Check sheet for the modelled part. Datum: model origin and axes. Units: mm. A direction names the side the tool comes from. Coordinates: 2 decimals unless noted, no trailing zeros. Loops run counter-clockwise (first coordinate to the right, second up) from the corner with the lowest first, then second, coordinate; pieces in that order, holes last.
from build123d import *

# Parameters (mm, degrees)
SKETCH1_R           = 32.75
BOSS_EXTRUDE1_DEPTH = 80.75
SKETCH12_R          = 6
BOSS_EXTRUDE5_DEPTH = 63
SKETCH13_R          = 2
CUT_EXTRUDE1_DEPTH  = 10
CIRPATTERN1_COUNT   = 6
SKETCH14_R          = 2.5
CUT_EXTRUDE2_DEPTH  = 10
CIRPATTERN2_COUNT   = 4


with BuildPart() as part:
    # Sketch1 → Boss-Extrude1 (new body, symmetric)
    with BuildSketch(Plane.XY):
        Circle(SKETCH1_R)
    extrude(amount=BOSS_EXTRUDE1_DEPTH, both=True)

    # Sketch10 → Revolve1 (revolve)
    with BuildSketch(Plane(origin=(0, 0, 0), x_dir=(0, 0, -1), z_dir=(1, 0, 0))):
        Polygon((-97.75, 0), (-97.75, 14), (-80.75, 19), (-80.75, 0), align=None)
    revolve(axis=Axis((0, 0, 1000), (0, 0, -1)))

    # Sketch12 → Boss-Extrude5 (add)
    with BuildSketch(Plane.XY.offset(97.75)):
        Circle(SKETCH12_R)
    extrude(amount=BOSS_EXTRUDE5_DEPTH)

    # Sketch13 → Cut-Extrude1 (cut)
    with BuildSketch(Plane.XY.offset(80.75)):
        with Locations((0, 21)):
            Circle(SKETCH13_R)
    cut_extrude1 = extrude(amount=-CUT_EXTRUDE1_DEPTH, mode=Mode.SUBTRACT)

    # CirPattern1: Cut-Extrude1 ×6 about axis
    cirpattern1_axis = Axis((0, 0, 0), (0, 0, 1))
    for i in range(1, CIRPATTERN1_COUNT):
        add(cut_extrude1.rotate(cirpattern1_axis, i * 360 / CIRPATTERN1_COUNT), mode=Mode.SUBTRACT)

    # Sketch14 → Cut-Extrude2 (cut)
    with BuildSketch(Plane(origin=(0, 0, -80.75), x_dir=(-1, 0, 0), z_dir=(0, 0, -1))):
        with Locations((14.849242405, 14.849242405)):
            Circle(SKETCH14_R)
    cut_extrude2 = extrude(amount=-CUT_EXTRUDE2_DEPTH, mode=Mode.SUBTRACT)

    # CirPattern2: Cut-Extrude2 ×4 about axis
    cirpattern2_axis = Axis((0, 0, 0), (0, 0, 1))
    for i in range(1, CIRPATTERN2_COUNT):
        add(cut_extrude2.rotate(cirpattern2_axis, i * 360 / CIRPATTERN2_COUNT), mode=Mode.SUBTRACT)


solid = part.part
(1) Set-up check for faces 1 (the face through (31.238, 9.837, 1.13)), 2 (the face through (0, 21, 70.75)), 3 (the face through (-13.89, -17.16, -75.82)): record each of +Z, -Z, +X, -X, +Y, -Y from which the full face is reachable in a straight line by a thin tool's end or side.
(2) Draft check along Y on faces 4 (the face through (-13.68, 7.12, 92.91)), 5 (the face through (18, -10, 70.75)), 6 (the face through (0, 0, -80.75)). Enter one of: pulls with the +Y half, pulls with the -Y half, needs draft (parallel to the pull), parting line crosses it, or undercut.
(3) Section check B-B, the plane z = 28. Enter the section's corners in (x, y), plus the area to 3 significant figures.
(4) Section check C-C, the plane z = 112. Enter the section's corners in (x, y), plus the area to 3 significant figures.
(5) Gauge pin test, flat ends, axial feed: P1, Ø1.5, axis at x = 14.5, z = 59.5, coming from the -Y side; P2, Ø2.5, axis at x = -14, y = -15, coming from the -Z side; P3, Ø1.5, axis at y = 0, z = 85, coming from the -X side. Record the tip position at first contact, or that the pin passes through.
(6) Section check A-A, the plane y = 0. Enter the section's corners in (x, z).
(7) Scan lines: line 1 along X through (y, z) = (10.5, 76); line 2 along X through (y, z) = (10, 75); line 3 along Z through (x, y) = (9.5, 22). Record each from-to range of solid material in increasing order.
Determined:
1. face 1: +Z, -Z
1. face 2: +Z
1. face 3: -Z
2. face 4: parting line crosses it
2. face 5: undercut
2. face 6: needs draft
3. outline: circle Ø65.5 at (0, 0)
3. area: 3,370 mm2
4. outline: circle Ø12 at (0, 0)
4. area: 113 mm2
5. P1: stops at y = -29.72
5. P2: stops at z = -70.75
5. P3: stops at x = -17.97
6. outline: (-32.75, -80.75) - (32.75, -80.75) - (32.75, 80.75) - (19, 80.75) - (14, 97.75) - (6, 97.75) - (6, 160.75) - (-6, 160.75) - (-6, 97.75) - (-14, 97.75) - (-19, 80.75) - (-32.75, 80.75) - close
7. line 1: x = -31.02 to -20.19, -16.19 to 16.19, 20.19 to 31.02
7. line 2: x = -31.19 to -20.12, -16.25 to 16.25, 20.12 to 31.19
7. line 3: z = -80.75 to 80.75
